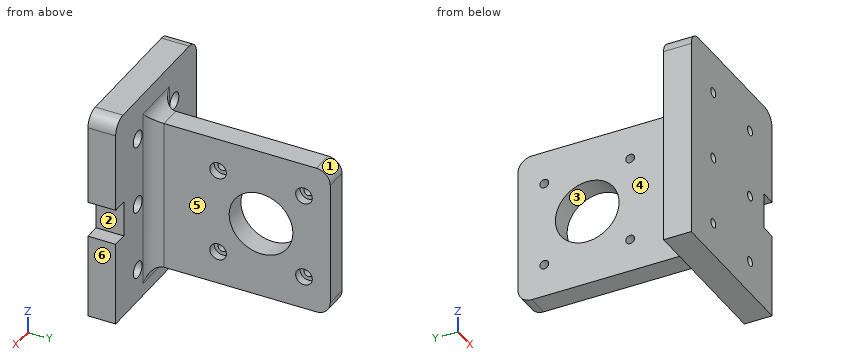
```python
from build123d import *

# Parameters (mm, degrees)
SKETCH1_W               = 55
SKETCH1_H               = 80
BOSS_EXTRUDE1_DEPTH     = 10
SKETCH6_R               = 1.65
CUT_EXTRUDE2_DEPTH      = 55
LPATTERN1_COUNT         = 3
LPATTERN1_PITCH         = 25
MIRROR3_COPY_1_SKETCH_R = 1.65
MIRROR3_COPY_1_DEPTH    = 55
MIRROR3_COPY_2_SKETCH_R = 1.65
MIRROR3_COPY_2_DEPTH    = 55
SKETCH8_W               = 8
SKETCH8_H               = 55
BOSS_EXTRUDE3_DEPTH     = 65
FILLET3_R               = 5
SKETCH9_R               = 1.6
SKETCH9_R_2             = 11.5
CUT_EXTRUDE3_DEPTH      = 32.5
SKETCH10_R              = 3
CUT_EXTRUDE4_DEPTH      = 3
CUT_EXTRUDE5_START      = -5
SKETCH11_R              = 3
CUT_EXTRUDE5_DEPTH      = 71
LPATTERN2_COUNT         = 3
LPATTERN2_PITCH         = 25
MIRROR4_START           = -5
MIRROR4_COPY_1_SKETCH_R = 3
MIRROR4_COPY_1_DEPTH    = 71
MIRROR4_COPY_2_SKETCH_R = 3
MIRROR4_COPY_2_DEPTH    = 71
SKETCH12_W              = 11
SKETCH12_H              = 13
CUT_EXTRUDE6_DEPTH      = 11
CUT_EXTRUDE7_DEPTH      = 10


with BuildPart() as part:
    # Sketch1 → Boss-Extrude1 (new body)
    with BuildSketch(Plane(origin=(0, 0, 0), x_dir=(1, 0, 0), z_dir=(0, 1, 0))):
        Rectangle(SKETCH1_W, SKETCH1_H)
    extrude(amount=BOSS_EXTRUDE1_DEPTH)

    # Sketch6 → Cut-Extrude2 (cut)
    with BuildSketch(Plane(origin=(0, 10, 0), x_dir=(1, 0, 0), z_dir=(0, 1, 0))):
        with Locations((-12.5, -25)):
            Circle(SKETCH6_R)
    cut_extrude2 = extrude(amount=-CUT_EXTRUDE2_DEPTH, mode=Mode.SUBTRACT)

    # LPattern1: Cut-Extrude2 ×3
    with Locations(*[(0, 0, -i * LPATTERN1_PITCH) for i in range(1, LPATTERN1_COUNT)]):
        add(cut_extrude2, mode=Mode.SUBTRACT)

    # Mirror3: Cut-Extrude2 across plane
    add(cut_extrude2.mirror(Plane(origin=(0, 0, 0), x_dir=(0, 0, 1), z_dir=(1, 0, 0))), mode=Mode.SUBTRACT)

    # Mirror3 copy 1 sketch → Mirror3 copy 1 (cut)
    with BuildSketch(Plane(origin=(0, 10, -25), x_dir=(-1, 0, 0), z_dir=(0, 1, 0))):
        with Locations((-12.5, 25)):
            Circle(MIRROR3_COPY_1_SKETCH_R)
    extrude(amount=-MIRROR3_COPY_1_DEPTH, mode=Mode.SUBTRACT)

    # Mirror3 copy 2 sketch → Mirror3 copy 2 (cut)
    with BuildSketch(Plane(origin=(0, 10, -50), x_dir=(-1, 0, 0), z_dir=(0, 1, 0))):
        with Locations((-12.5, 25)):
            Circle(MIRROR3_COPY_2_SKETCH_R)
    extrude(amount=-MIRROR3_COPY_2_DEPTH, mode=Mode.SUBTRACT)

    # Sketch8 → Boss-Extrude3 (add)
    with BuildSketch(Plane(origin=(0, 10, 0), x_dir=(1, 0, 0), z_dir=(0, 1, 0))):
        Rectangle(SKETCH8_W, SKETCH8_H)
    extrude(amount=BOSS_EXTRUDE3_DEPTH)

    # Fillet3
    fillet3_edges = [part.edges().sort_by_distance(p)[0] for p in [
        (4, 10, 0),
        (0, 10, -27.5),
        (-4, 10, 0),
        (0, 10, 27.5),
        (0, 75, -27.5),
        (0, 75, 27.5),
        (27.5, 5, 40),
        (-27.5, 5, 40),
    ]]
    fillet(fillet3_edges, radius=FILLET3_R)

    # Sketch9 → Cut-Extrude3 (cut, through all)
    with BuildSketch(Plane.ZY.offset(4)):
        with Locations((-15.5, 65.5)):
            Circle(SKETCH9_R)
        with Locations((15.5, 65.5)):
            Circle(SKETCH9_R)
        with Locations((-15.5, 34.5)):
            Circle(SKETCH9_R)
        with Locations((15.5, 34.5)):
            Circle(SKETCH9_R)
        with Locations((0, 50)):
            Circle(SKETCH9_R_2)
    extrude(amount=-CUT_EXTRUDE3_DEPTH, mode=Mode.SUBTRACT)

    # Sketch10 → Cut-Extrude4 (cut)
    with BuildSketch(Plane(origin=(4, 0, 0), x_dir=(0, 0, -1), z_dir=(1, 0, 0))):
        with Locations((-15.5, 65.5)):
            Circle(SKETCH10_R)
        with Locations((15.5, 65.5)):
            Circle(SKETCH10_R)
        with Locations((15.5, 34.5)):
            Circle(SKETCH10_R)
        with Locations((-15.5, 34.5)):
            Circle(SKETCH10_R)
    extrude(amount=-CUT_EXTRUDE4_DEPTH, mode=Mode.SUBTRACT)

    # Sketch11 → Cut-Extrude5 (cut)
    with BuildSketch(Plane(origin=(0, 10, 0), x_dir=(1, 0, 0), z_dir=(0, 1, 0)).offset(CUT_EXTRUDE5_START)):
        with Locations((-12.5, -25)):
            Circle(SKETCH11_R)
    cut_extrude5 = extrude(amount=CUT_EXTRUDE5_DEPTH, mode=Mode.SUBTRACT)

    # LPattern2: Cut-Extrude5 ×3
    with Locations(*[(0, 0, -i * LPATTERN2_PITCH) for i in range(1, LPATTERN2_COUNT)]):
        add(cut_extrude5, mode=Mode.SUBTRACT)

    # Mirror4: Cut-Extrude5 across plane
    add(cut_extrude5.mirror(Plane(origin=(0, 0, 0), x_dir=(0, 0, 1), z_dir=(1, 0, 0))), mode=Mode.SUBTRACT)

    # Mirror4 copy 1 sketch → Mirror4 copy 1 (cut)
    with BuildSketch(Plane(origin=(0, 10, -25), x_dir=(-1, 0, 0), z_dir=(0, 1, 0)).offset(MIRROR4_START)):
        with Locations((-12.5, 25)):
            Circle(MIRROR4_COPY_1_SKETCH_R)
    extrude(amount=MIRROR4_COPY_1_DEPTH, mode=Mode.SUBTRACT)

    # Mirror4 copy 2 sketch → Mirror4 copy 2 (cut)
    with BuildSketch(Plane(origin=(0, 10, -50), x_dir=(-1, 0, 0), z_dir=(0, 1, 0)).offset(MIRROR4_START)):
        with Locations((-12.5, 25)):
            Circle(MIRROR4_COPY_2_SKETCH_R)
    extrude(amount=MIRROR4_COPY_2_DEPTH, mode=Mode.SUBTRACT)

    # Sketch12 → Cut-Extrude6 (cut, through all)
    with BuildSketch(Plane(origin=(0, 10, 0), x_dir=(1, 0, 0), z_dir=(0, 1, 0))):
        with Locations((27.5, 0)):
            Rectangle(SKETCH12_W, SKETCH12_H)
    extrude(amount=-CUT_EXTRUDE6_DEPTH, mode=Mode.SUBTRACT)

    # Sketch13 → Cut-Extrude7 (cut)
    with BuildSketch(Plane(origin=(0, 10, 0), x_dir=(1, 0, 0), z_dir=(0, 1, 0))):
        Polygon((-12.5, 37), (34.859752384, 37), (34.859752384, 45.853513443), (-44.482070636, 45.853513443), (-44.482070636, 37), align=None)
    extrude(amount=-CUT_EXTRUDE7_DEPTH, mode=Mode.SUBTRACT)


solid = part.part
```
Here's how the part is built. I have some questions about the finished solid (model axes, mm). Face numbers are marked on the shaded views. A direction names the side the tool comes from. Coordinates: 2 decimals unless noted, no trailing zeros. Loops run counter-clockwise (first coordinate to the right, second up) from the corner with the lowest first, then second, coordinate; pieces in that order, holes last. Notation, with made-up numbers: M 56.5,-35.75 L 70.5,-35.75 A27 cw 70.5,3.25 Z; hole C 36.25,67.5 d10. An arc over 180 degrees is marked long. One line per item, written item: value.
1. On a 3-axis mill with a long thin cutter (end or side, diameter ignored), from which of +Z, -Z, +X, -X, +Y, -Y can I reach the whole of each face in a straight line? I mean the marked faces 5 and 6. Say none if no direction works.
Geometry says:
face 5: +Z, -Z, +X, +Y
face 6: +Z, -Z, +X, +Y, -Y
2. Imagine slicing it at A-A (z = 0). State how many separate pieces and enclosed holes the cut face has, and give its area (3 significant figures).
Geometry says:
separate pieces: 4
enclosed holes: 0
area: 749 mm2
3. Please list where these lines run through material, in increasing order: probe 1 along Z at (x, y) = (-1.8, 65.5); probe 2 along Z at (x, y) = (-12.5, 8.65); probe 3 along Z at (x, y) = (12.5, 1.6).
Geometry says:
probe 1: z = -27.5 to -17.1, -13.9 to 13.9, 17.1 to 27.5
probe 2: z = -37 to -28, -22 to -3, 3 to 22, 28 to 40
probe 3: z = -37 to -26.65, -23.35 to -1.65, 1.65 to 23.35, 26.65 to 40
4. Imagine slicing it at C-C (z = 15.5). List the corners of the cut face in (x, y) for me.
Geometry says:
outline: M -27.5,0 L 27.5,0 L 27.5,10 L 9,10 A5 cw 4,15 L 4,31.5 L 1,31.5 L 1,32.9 L -4,32.9 L -4,15 A5 cw -9,10 L -27.5,10 Z; M -4,36.1 L 1,36.1 L 1,37.5 L 4,37.5 L 4,62.5 L 1,62.5 L 1,63.9 L -4,63.9 Z; M -4,67.1 L 1,67.1 L 1,68.5 L 4,68.5 L 4,75 L -4,75 Z
5. Imagine slicing it at D-D (x = -12.5). List the corners of the cut face in (y, z) for me, and give its area (4 significant figures).
Geometry says:
outline: M 0,-37 L 10,-37 L 10,-28 L 5,-28 L 5,-26.65 L 0,-26.65 Z; M 0,-23.35 L 5,-23.35 L 5,-22 L 10,-22 L 10,-3 L 5,-3 L 5,-1.65 L 0,-1.65 Z; M 0,1.65 L 5,1.65 L 5,3 L 10,3 L 10,22 L 5,22 L 5,23.35 L 0,23.35 Z; M 0,26.65 L 5,26.65 L 5,28 L 10,28 L 10,40 L 0,40 Z
area: 630.5 mm2
6. Will these pins go through, and if not, where does the flat tip stop? pin 1 Ø1.8 at (x, z) = (-12, 1.5) entering from +Y; pin 2 Ø1.8 at (x, z) = (12.5, 0) entering from +Y; pin 3 Ø10 at (x, y) = (7, 26) entering from +Z; pin 4 Ø10 at (x, y) = (-8.5, 39.5) entering from -Z.
Geometry says:
pin 1: stops at y = 5
pin 2: passes through
pin 3: stops at z = 27.5
pin 4: stops at z = -27.5
7. Imagine slicing it at B-B (y = 65.5). List the corners of the cut face in (x, z) for me.
Geometry says:
outline: M -4,-27.5 L 4,-27.5 L 4,-18.5 L 1,-18.5 L 1,-17.1 L -4,-17.1 Z; M -4,-13.9 L 1,-13.9 L 1,-12.5 L 4,-12.5 L 4,12.5 L 1,12.5 L 1,13.9 L -4,13.9 Z; M -4,17.1 L 1,17.1 L 1,18.5 L 4,18.5 L 4,27.5 L -4,27.5 Z
8. Thinking about a two-plate mould opening in Z: for the marked faces 1, 2, 3 and 4, which applies, +Z half, -Z half, draft (parallel to the pull), parting line (faces both ways), or undercut?
Geometry says:
face 1: +Z half
face 2: undercut
face 3: undercut
face 4: draft
